```python
from build123d import *

# Parameters (mm, degrees)
SKETCH1_W            = 50.8
SKETCH1_H            = 30
SKETCH1_R            = 4
BOSS_EXTRUDE1_DEPTH  = 25.4
SKETCH2_R            = 4
BOSS_EXTRUDE3_DEPTH  = 50.8
SKETCH4_W            = 25.4
SKETCH4_H            = 10
BOSS_EXTRUDE4_DEPTH  = 19.3499994
M4_CLEARANCE_HOLE1_D = 4.5


with BuildPart() as part:
    # Sketch1 → Boss-Extrude1 (new body)
    with BuildSketch(Plane.XY):
        with Locations((0, -9)):
            Rectangle(SKETCH1_W, SKETCH1_H)
        Circle(SKETCH1_R, mode=Mode.SUBTRACT)
    extrude(amount=BOSS_EXTRUDE1_DEPTH)

    # Sketch2 → Boss-Extrude3 (add, through all)
    with BuildSketch(Plane(origin=(25.4, 0, 0), x_dir=(0, 0, -1), z_dir=(1, 0, 0))):
        with BuildLine():
            Line((-25.4, 6), (-25.4, 5))
            Line((-25.4, 5), (0, 5))
            Line((0, 5), (0, 6))
            ThreePointArc((0, 6), (-12.7, 18.7), (-25.4, 6))
        make_face()
        with Locations(Location((-12.7, 10, 0), (0, 0, 90))):
            Circle(SKETCH2_R, mode=Mode.SUBTRACT)
    extrude(amount=-BOSS_EXTRUDE3_DEPTH)

    # Sketch4 → Boss-Extrude4 (add)
    with BuildSketch(Plane.ZY.offset(25.4)):
        with Locations((12.7, -4)):
            Rectangle(SKETCH4_W, SKETCH4_H)
    extrude(amount=BOSS_EXTRUDE4_DEPTH)

    # M4 Clearance Hole1 (through all)
    with Locations(Plane(origin=(0, -9, 0), x_dir=(-1, 0, 0), z_dir=(0, -1, 0))):
        with Locations((35.0749997, -12.7)):
            Hole(M4_CLEARANCE_HOLE1_D / 2)


solid = part.part
```
Model file for the job. Use its own axes, mm. A direction names the side the tool comes from. Give positions to 0.01 mm unless a question says otherwise; leave off trailing zeros. Loops run counter-clockwise (first coordinate to the right, second up) from the corner with the lowest first, then second, coordinate; pieces in that order, holes last. Notation, with made-up numbers: (-21.75, 48.5) -> (22.25, 48.5) arc R6 cw to (22.25, 52.5) -> close; hole circle Ø1 at (-27, 23). An arc over 180 degrees is marked (long way). Use CSV: the item, a comma, the result in double quotes. Start each with the question number.
1) Slice it at B-B on y = 0. Give the cut face in (x, z) (3 decimals), plus the area to 3 significant figures.
2) Flat gauge pins, fed straight in: pin 1 Ø6 at (x, z) = (10.5, 22.5) entering from +Y; pin 2 Ø7.5 at (y, z) = (-18, 14.5) entering from -X; pin 3 Ø9.5 at (x, z) = (-35, 8.5) entering from +Y; pin 4 Ø1 at (x, y) = (-13, -9.5) entering from -Z. Where does each tip first touch, or does it go through?
3) Slice it at A-A on z = 12.7. Give the cut face in (x, y) (3 decimals), plus the area to 3 significant figures.
4) Mould opens along Z. For faces 4 (the cylindrical face through (0.4, 6.8, 10.3)), 5 (the cylindrical face through (-37.323, -3.93, 12.601)), 6 (the cylindrical face through (0.356, 18.697, 12.421)), 7 (the flat face through (0, -24, 13)) say: released by +Z, released by -Z, zero draft, split by the parting line, or undercut.
5) Slice it at C-C on x = 0. Give the cut face in (y, z).
6) Tool access for faces 1 (the flat face through (-44.75, -4, 13)), 2 (the flat face through (-34.9, -9, 15.3)), 3 (the flat face through (-34.9, 1, 15.3)): list every direction of +Z, -Z, +X, -X, +Y, -Y with a clear straight run to the whole face (end or side of a thin tool).
7) Wall check: line 1 (X direction, y = -5, z = 12.7) (3 decimals); line 2 (Y direction, x = 0, z = 10.5); line 3 (X direction, y = -10, z = 14). Give the ranges that are in metal, low to high.
8) Slice it at D-D on z = 16. Give the cut face in (x, y).
Computed values:
1,outline,"(-44.75, 0) -> (-4, 0) -> (-4, 25.4) -> (-44.75, 25.4) -> close; (4, 0) -> (25.4, 0) -> (25.4, 25.4) -> (4, 25.4) -> close; hole circle Ø4.5 at (-35.075, 12.7)"
1,area,"1,560 mm^2"
2,pin 1,"stops at y = 16.73"
2,pin 2,"stops at x = -25.4"
2,pin 3,"stops at y = 1"
2,pin 4,"stops at z = 0"
3,outline,"(-44.75, -9) -> (-37.325, -9) -> (-37.325, 1) -> (-44.75, 1) -> close; (-32.825, -9) -> (-25.4, -9) -> (-25.4, -24) -> (25.4, -24) -> (25.4, 6) -> (-25.4, 6) -> (-25.4, 1) -> (-32.825, 1) -> close; (-25.4, 14) -> (25.4, 14) -> (25.4, 18.7) -> (-25.4, 18.7) -> close; hole circle Ø8 at (0, 0)"
3,area,"1,860 mm^2"
4,face 4,"undercut"
4,face 5,"undercut"
4,face 6,"split by the parting line"
4,face 7,"zero draft"
5,outline,"(-24, 0) -> (-4, 0) -> (-4, 25.4) -> (-24, 25.4) -> close; (4, 0) -> (6, 0) arc R12.7 ccw to (6, 25.4) -> (4, 25.4) -> close; hole circle Ø8 at (10, 12.7)"
6,face 1,"+Z, -Z, -X, +Y, -Y"
6,face 2,"+Z, -Z, -X, -Y"
6,face 3,"+Z, -Z, -X, +Y"
7,line 1,"x = -44.75 to -37.325, -32.825 to 25.4"
7,line 2,"y = -24 to -4, 4 to 6.66, 13.34 to 18.51"
7,line 3,"x = -25.4 to 25.4"
8,outline,"(-44.75, -9) -> (-25.4, -9) -> (-25.4, -24) -> (25.4, -24) -> (25.4, 7.74) -> (-25.4, 7.74) -> (-25.4, 1) -> (-44.75, 1) -> close; (-25.4, 12.26) -> (25.4, 12.26) -> (25.4, 18.26) -> (-25.4, 18.26) -> close; hole circle Ø8 at (0, 0)"
